```python
from build123d import *

# Parameters (mm, degrees)
SKETCH1_W           = 26
SKETCH1_H           = 22.12
SKETCH1_R           = 1.75
BOSS_EXTRUDE1_DEPTH = 5.13
CUT_EXTRUDE1_REACH  = 28.165
SKETCH2_R           = 1.5
BOSS_EXTRUDE2_DEPTH = 3


with BuildPart() as part:
    # Sketch1 → Boss-Extrude1 (new body)
    with BuildSketch(Plane(origin=(0, 0, 0), x_dir=(1, 0, 0), z_dir=(0, 1, 0))):
        Rectangle(SKETCH1_W, SKETCH1_H)
        with Locations(Location((6.25, -5, 0), (0, 0, 270))):
            Circle(SKETCH1_R, mode=Mode.SUBTRACT)
        with Locations(Location((-6.25, -5, 0), (0, 0, 270))):
            Circle(SKETCH1_R, mode=Mode.SUBTRACT)
        with Locations(Location((-6.25, 5, 0), (0, 0, 270))):
            Circle(SKETCH1_R, mode=Mode.SUBTRACT)
        with Locations(Location((6.25, 5, 0), (0, 0, 270))):
            Circle(SKETCH1_R, mode=Mode.SUBTRACT)
    extrude(amount=BOSS_EXTRUDE1_DEPTH)

    # Sketch2 → Cut-Extrude1 (cut, up to next)
    with BuildSketch(Plane.XY.offset(11.06), mode=Mode.PRIVATE) as cut_extrude1_sk1:
        with Locations((0, 2.565)):
            Circle(SKETCH2_R)
    cut_extrude1_tool1 = extrude(cut_extrude1_sk1.sketch, amount=-CUT_EXTRUDE1_REACH, mode=Mode.PRIVATE) & part.part
    # Sketch2 → Cut-Extrude1 (cut, up to next)
    with BuildSketch(Plane.XY.offset(11.06), mode=Mode.PRIVATE) as cut_extrude1_sk2:
        with Locations((-10, 2.565)):
            Circle(SKETCH2_R)
    cut_extrude1_tool2 = extrude(cut_extrude1_sk2.sketch, amount=-CUT_EXTRUDE1_REACH, mode=Mode.PRIVATE) & part.part
    # Sketch2 → Cut-Extrude1 (cut, up to next)
    with BuildSketch(Plane.XY.offset(11.06), mode=Mode.PRIVATE) as cut_extrude1_sk3:
        with Locations(Location((10, 2.565, 0), (0, 0, 180))):
            Circle(SKETCH2_R)
    cut_extrude1_tool3 = extrude(cut_extrude1_sk3.sketch, amount=-CUT_EXTRUDE1_REACH, mode=Mode.PRIVATE) & part.part
    add(cut_extrude1_tool1.solids().sort_by_distance((0, 2.565, 11.06))[0], mode=Mode.SUBTRACT)
    add(cut_extrude1_tool2.solids().sort_by_distance((-10, 2.565, 11.06))[0], mode=Mode.SUBTRACT)
    add(cut_extrude1_tool3.solids().sort_by_distance((10, 2.565, 11.06))[0], mode=Mode.SUBTRACT)

    # Sketch3 → Boss-Extrude2 (add)
    with BuildSketch(Plane.XZ):
        with BuildLine():
            Line((-13, -11.06), (-11.035, -11.06))
            Line((-11.035, -11.06), (-11.63, 2.57))
            add(Edge.make_bspline(
                [(-11.63, 2.57), (-11.34945273, 3.758467492), (-10.92, 4.9)],
                knots=[0, 0, 0, 1, 1, 1], degree=2))
            Line((-10.92, 4.9), (-7.881497006, 11.06))
            Line((-7.881497006, 11.06), (-13, 11.06))
            Line((-13, 11.06), (-13, -11.06))
        make_face()
        with BuildLine():
            Line((11.63, 2.57), (11.035, -11.06))
            Line((11.035, -11.06), (13, -11.06))
            Line((13, -11.06), (13, 11.06))
            Line((13, 11.06), (7.881497006, 11.06))
            Line((7.881497006, 11.06), (10.92, 4.9))
            add(Edge.make_bspline(
                [(11.63, 2.57), (11.34945273, 3.758467492), (10.92, 4.9)],
                knots=[0, 0, 0, 1, 1, 1], degree=2))
        make_face()
    extrude(amount=BOSS_EXTRUDE2_DEPTH)


solid = part.part
```
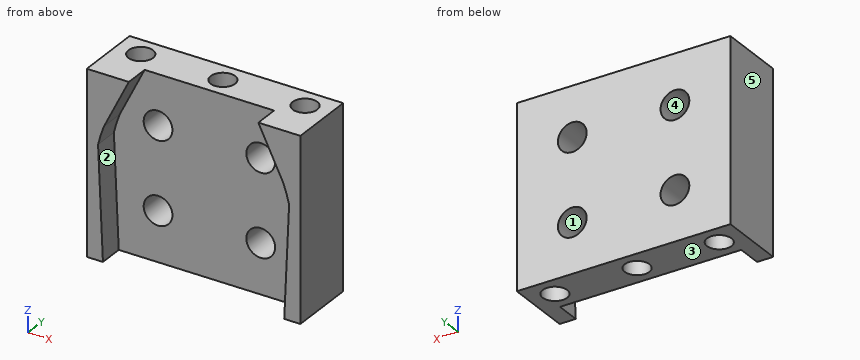
Geometry check sheet. Reference: the model listing, model coordinates, mm. Face numbers are marked on the shaded views. A direction names the side the tool comes from. Coordinates: 2 decimals unless noted, no trailing zeros. Write each loop counter-clockwise with the first axis right and the second up, starting at its lowest first coordinate (ties: lowest second). Pieces come first, ordered by that corner, then holes. Notation, with made-up numbers: M -36,-0.5 L -15,-0.5 A22 ccw -15,23.5 Z; hole C 74.25,13.25 d5. An arc over 180 degrees is marked long. One line per item, written item: value. Start each with the question number.
(1) Scan lines: line 1 along X through (y, z) = (3.75, -1.75); line 2 along X through (y, z) = (3.25, 2); line 3 along Y through (x, z) = (1, 10.25). Record each from-to range of solid material in increasing order. Write a range as [from, to].
(2) Release check for a two-part mould opening along X. For the marked faces 3, 4 and 5 record: released by +X, released by -X, zero draft, split by the parting line, or undercut.
(3) Tool access check on the marked faces 1 and 2. Record the directions out of +Z, -Z, +X, -X, +Y, -Y that give a thin tool (end or side, any length) a straight path to the whole face; none if there is none.
(4) Sectioned sample at D-D, the plane x = 6.25. Enter the section's corners in (y, z).
(5) Depth check by flat-ended pin: pin 1 (1 mm diameter, centred on x = -3.5, z = 6.5, fed in from -Y). Enter the tip coordinate at first touch or a pass-through.
(6) Sectioned sample at C-C, the plane z = -5. Enter the section's corners in (x, y) (3 decimals).
(7) Sectioned sample at A-A, the plane x = 0. Enter the section's corners in (y, z) (3 decimals), and give its area (3 significant figures).
(8) Sectioned sample at B-B, the plane y = 1.5. Enter the section's corners in (x, z).
Filled sheet:
1. line 1: [-13, -10.92], [-9.08, -0.92], [0.92, 9.08], [10.92, 13]
1. line 2: [-13, -11.33], [-8.67, -1.33], [1.33, 8.67], [11.33, 13]
1. line 3: [0, 1.45], [3.68, 5.13]
2. face 3: zero draft
2. face 4: undercut
2. face 5: released by -X
3. face 1: +Y, -Y
3. face 2: -Y
4. outline: M 0,-11.06 L 5.13,-11.06 L 5.13,-6.75 L 0,-6.75 Z; M 0,-3.25 L 5.13,-3.25 L 5.13,3.25 L 0,3.25 Z; M 0,6.75 L 5.13,6.75 L 5.13,11.06 L 0,11.06 Z
5. pin 1: y = 0
6. outline: M -13,-3 L -11.3,-3 L -11.3,0 L -8,0 L -8,5.13 L -13,5.13 Z; M -4.5,0 L 4.5,0 L 4.5,5.13 L -4.5,5.13 Z; M 8,0 L 11.3,0 L 11.3,-3 L 13,-3 L 13,5.13 L 8,5.13 Z; hole C -10,2.565 d3; hole C 0,2.565 d3; hole C 10,2.565 d3
7. outline: M 0,-11.06 L 1.065,-11.06 L 1.065,11.06 L 0,11.06 Z; M 4.065,-11.06 L 5.13,-11.06 L 5.13,11.06 L 4.065,11.06 Z
7. area: 47.1 mm²
8. outline: M -13,-11.06 L -11.06,-11.06 L -11.06,11.06 L -13,11.06 Z; M -8.94,-11.06 L -1.06,-11.06 L -1.06,11.06 L -8.94,11.06 Z; M 1.06,-11.06 L 8.94,-11.06 L 8.94,11.06 L 1.06,11.06 Z; M 11.06,-11.06 L 13,-11.06 L 13,11.06 L 11.06,11.06 Z; hole C -6.25,-5 d3.5; hole C -6.25,5 d3.5; hole C 6.25,-5 d3.5; hole C 6.25,5 d3.5
